Geometry: final body of the model. Coordinates: model frame, mm. Give positions to 0.01 mm unless a question says otherwise; leave off trailing zeros. Write each loop counter-clockwise with the first axis right and the second up, starting at its lowest first coordinate (ties: lowest second). Pieces come first, ordered by that corner, then holes. Notation, with made-up numbers: M 25,-7 L 36,-7 A29 cw 36,23 Z; hole C 10,36.25 d5. An arc over 180 degrees is marked long. Use one line per item in the form item = value. Start each with the question number.
Item 1: Section query A-A on x = 0. Return loops of the section in (y, z) (3 decimals).
Item 2: Section query B-B on y = -143.65. Return loops of the section in (x, z) (3 decimals).
Item 3: Section query D-D on y = 47.5. Return loops of the section in (x, z) (3 decimals), then the cut area to 3 significant figures.
Item 4: Material intervals for line 1 along Y through (x, z) = (-12, 0.75); line 2 along X through (y, z) = (110, 0.25); line 3 along Y through (x, z) = (-9.5, 2.75), sorted ascending. Write a range as from..to.
Item 5: Contact query for flat-ended pins moving along their axis: P1, Ø2, axis at y = 71.5, z = -2.5, coming from the +X side; P2, Ø4, axis at x = 0, y = -143.65, coming from the -Z side; P3, Ø1.9, axis at x = 14, z = 1.5, coming from the -Y side; P4, Ø2, axis at y = 61, z = 2.5, coming from the -X side. Output: stop coordinate, or through.
Item 6: Section query C-C on z = 0.75. Return loops of the section in (x, y) (3 decimals), then the cut area to 3 significant figures.
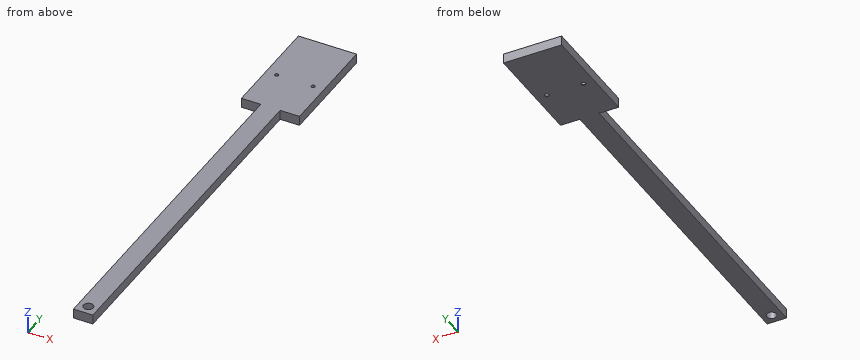
from build123d import *

# Parameters (mm, degrees)
CROQUIS1_W                      = 12.7
CROQUIS1_H                      = 6.35
SALIENTE_EXTRUIR1_DEPTH         = 150
CORTAR_EXTRUIR1_DEPTH           = 151.16791643
CORTAR_EXTRUIR1_DEPTH_BACK      = 151.16791643
CROQUIS2_R                      = 3.175
CROQUIS3_W                      = 38.1
CROQUIS3_H                      = 6.35
SALIENTE_EXTRUIR2_DEPTH         = 70
TALADRO_ROSCADO_M31_D           = 2.5
TALADRO_ROSCADO_M31_CSINK_D     = 3.05
TALADRO_ROSCADO_M31_CSINK_ANGLE = 90


with BuildPart() as part:
    # Croquis1 → Saliente-Extruir1 (new, symmetric)
    with BuildSketch(Plane(origin=(0, 0, 0), x_dir=(1, 0, 0), z_dir=(0, 1, 0))):
        Rectangle(CROQUIS1_W, CROQUIS1_H)
    extrude(amount=SALIENTE_EXTRUIR1_DEPTH, both=True)

    # Croquis2 → Cortar-Extruir1 (cut, two sides: drawn at the far end of the back side and taken through both)
    with BuildSketch(Plane.XY.offset(-CORTAR_EXTRUIR1_DEPTH_BACK)):
        with Locations((0, -143.65)):
            Circle(CROQUIS2_R)
    extrude(amount=CORTAR_EXTRUIR1_DEPTH + CORTAR_EXTRUIR1_DEPTH_BACK, mode=Mode.SUBTRACT)

    # Croquis3 → Saliente-Extruir2 (add)
    with BuildSketch(Plane(origin=(0, 150, 0), x_dir=(1, 0, 0), z_dir=(0, 1, 0))):
        Rectangle(CROQUIS3_W, CROQUIS3_H)
    extrude(amount=-SALIENTE_EXTRUIR2_DEPTH)

    # Taladro roscado M31 (through all)
    with Locations(Plane(origin=(0, 0, -3.175), x_dir=(-1, 0, 0), z_dir=(0, 0, -1))):
        with Locations((12, 110), (-12, 110)):
            CounterSinkHole(TALADRO_ROSCADO_M31_D / 2, TALADRO_ROSCADO_M31_CSINK_D / 2, counter_sink_angle=TALADRO_ROSCADO_M31_CSINK_ANGLE)


solid = part.part
Answer sheet:
q1.outline = M -150,-3.175 L -146.825,-3.175 L -146.825,3.175 L -150,3.175 Z; M -140.475,-3.175 L 150,-3.175 L 150,3.175 L -140.475,3.175 Z
q2.outline = M -6.35,-3.175 L -3.175,-3.175 L -3.175,3.175 L -6.35,3.175 Z; M 3.175,-3.175 L 6.35,-3.175 L 6.35,3.175 L 3.175,3.175 Z
q3.outline = M -6.35,-3.175 L 6.35,-3.175 L 6.35,3.175 L -6.35,3.175 Z
q3.area = 80.6 mm2
q4.line_1 = 80..108.75, 111.25..150
q4.line_2 = -19.05..-13.25, -10.75..10.75, 13.25..19.05
q4.line_3 = 80..150
q5.P1 = 6.35
q5.P2 = through
q5.P3 = 80
q5.P4 = -6.35
q6.outline = M -19.05,80 L -6.35,80 L -6.35,-150 L 6.35,-150 L 6.35,80 L 19.05,80 L 19.05,150 L -19.05,150 Z; hole C -12,110 d2.5; hole C 0,-143.65 d6.35; hole C 12,110 d2.5
q6.area = 5,550 mm2
